Part model, mm, in its own coordinate system. A direction names the side the tool comes from. Coordinates: 2 decimals unless noted, no trailing zeros. Order: outer loops, then holes, each group sorted by start corner. A loop starts at its lowest first (then second) coordinate and runs counter-clockwise, first axis right, second up.
from build123d import *

# Parameters (mm, degrees)
SZKIC1_R                          = 14
SZKIC1_R_2                        = 11.5
WYCI_GNI_CIE_CIENKA_CIANKA1_DEPTH = 1.5
SZKIC2_R                          = 11.5
SZKIC2_R_2                        = 10
DODANIE_WYCI_GNI_CIE1_DEPTH       = 15
ZAOKR_GLENIE1_R                   = 0.5
SFAZOWANIE1_SIZE                  = 0.8
SFAZOWANIE1_SIZE2                 = 0.461880215


with BuildPart() as part:
    # Szkic1 → Wyciągnięcie-cienka ścianka1 (new body)
    with BuildSketch(Plane.XY):
        Circle(SZKIC1_R)
        Circle(SZKIC1_R_2, mode=Mode.SUBTRACT)
    extrude(amount=WYCI_GNI_CIE_CIENKA_CIANKA1_DEPTH)

    # Szkic2 → Dodanie-wyciągnięcie1 (add)
    with BuildSketch(Plane.XY):
        Circle(SZKIC2_R)
        Circle(SZKIC2_R_2, mode=Mode.SUBTRACT)
    extrude(amount=DODANIE_WYCI_GNI_CIE1_DEPTH)

    # Zaokrąglenie1
    zaokr_glenie1_edges = [part.edges().sort_by_distance(p)[0] for p in [
        (-11.5, 0, 1.5),
    ]]
    fillet(zaokr_glenie1_edges, radius=ZAOKR_GLENIE1_R)

    # Sfazowanie1
    sfazowanie1_edges = [part.edges().sort_by_distance(p)[0] for p in [
        (-11.5, 0, 15),
    ]]
    sfazowanie1_side = [part.faces().sort_by_distance(p)[0] for p in [
        (-11.5, 0, 8.5),
    ]]
    chamfer(sfazowanie1_edges, length=SFAZOWANIE1_SIZE, length2=SFAZOWANIE1_SIZE2, reference=sfazowanie1_side[0])


solid = part.part
Q1. Pin check, flat tips, straight feed: pin 1 Ø5 at (y, z) = (8, 10) entering from +X; pin 2 Ø5 at (y, z) = (-1.5, 9) entering from -X; pin 3 Ø5 at (x, z) = (2.5, 2.5) entering from +Y; pin 4 Ø8 at (x, z) = (-9, 6.5) entering from -Y. Stop position of each tip, or through.
Results list:
pin 1: stops at x = 10.1
pin 2: stops at x = -11.5
pin 3: stops at y = 14
pin 4: stops at y = -10.36
Q2. Wall check: line 1 along Y through (x, z) = (0, 9); line 2 along Y through (x, z) = (8.75, 11.25); line 3 along Z through (x, y) = (-6, 11.25). Give the ranges that are in metal, low to high.
Results list:
line 1: y = -11.5 to -10, 10 to 11.5
line 2: y = -7.46 to -4.84, 4.84 to 7.46
line 3: z = 0 to 1.5
Q3. Cut at A-A on x = 0. Write the cut outline in (y, z).
Results list:
outline: (-14, 0) - (-10, 0) - (-10, 15) - (-11.04, 15) - (-11.5, 14.2) - (-11.5, 2) arc R0.5 cw to (-12, 1.5) - (-14, 1.5) - close; (10, 0) - (14, 0) - (14, 1.5) - (12, 1.5) arc R0.5 cw to (11.5, 2) - (11.5, 14.2) - (11.04, 15) - (10, 15) - close
Q4. Which spindle directions (+Z, -Z, +X, -X, +Y, -Y) get a long thin tool onto all of the face, cutting with end or side? Do faces 1 (the face through (-6.3, 10.4, 1.5)), 2 (the face through (-3, 10, 0)). Say none if no direction does.
Results list:
face 1: +Z
face 2: -Z, +X, -X, +Y, -Y
Q5. Mould opens along Y. For faces 3 (the face through (-2.17, -9.76, 7.4)), 4 (the face through (-2, 10, 15)), 5 (the face through (12.932, -5.362, 0.74)) say: pulls with the +Y half, pulls with the -Y half, needs draft (parallel to the pull), parting line crosses it, or undercut.
Results list:
face 3: undercut
face 4: needs draft
face 5: parting line crosses it
Q6. Cut at C-C on z = 13.5. Write the cut outline in (x, y).
Results list:
outline: circle Ø23 at (0, 0); hole circle Ø20 at (0, 0)
